Verification items for this drawing (mm, ordinates from the low corner). A direction names the side the tool comes from. Round coordinates to 2 decimals unless told otherwise and drop trailing zeros. Order: outer loops, then holes, each group sorted by start corner. A loop starts at its lowest first (then second) coordinate and runs counter-clockwise, first axis right, second up. Notation, with made-up numbers: (31.25, -9.75) -> (41.25, -9.75) arc R18 ccw to (41.25, 18.25) -> close; hole circle Ø5 at (66.5, -10). An arc over 180 degrees is marked (long way). Use a Markdown table: item, result. Add a question column.
Item 1: Sectioned sample at A-A, the plane z = 61. Record the cut outline in (x, y), and give its area (3 significant figures).
Item 2: Set-up check for the marked faces 1, 2 and 3: record each of +Z, -Z, +X, -X, +Y, -Y from which the full face is reachable in a straight line by a thin tool's end or side.
Item 3: Sectioned sample at D-D, the plane z = 270. Record the cut outline in (x, y), and give its area (3 significant figures).
Item 4: Gauge pin test, flat ends, axial feed: pin 1 Ø4 at (x, y) = (56.5, 411) entering from -Z; pin 2 Ø12 at (x, y) = (221, 991.5) entering from +Z; pin 3 Ø12 at (x, y) = (143.5, 2277.5) entering from +Z; pin 4 Ø4 at (y, z) = (1133, 263.5) entering from -X. Record the tip position at first contact, or that the pin passes through.
Item 5: Sectioned sample at B-B, the plane x = 207.5. Record the cut outline in (y, z).
Item 6: Material ranges on probe 1 along X at (y, z) = (819, 104); probe 2 along Y at (x, z) = (229, 436.5); probe 3 along Z at (x, y) = (203.5, 303), recorded low to high. Write a range as [from, to].
Item 7: Sectioned sample at C-C, the plane y = 1834. Record the cut outline in (x, z), and give its area (3 significant figures).
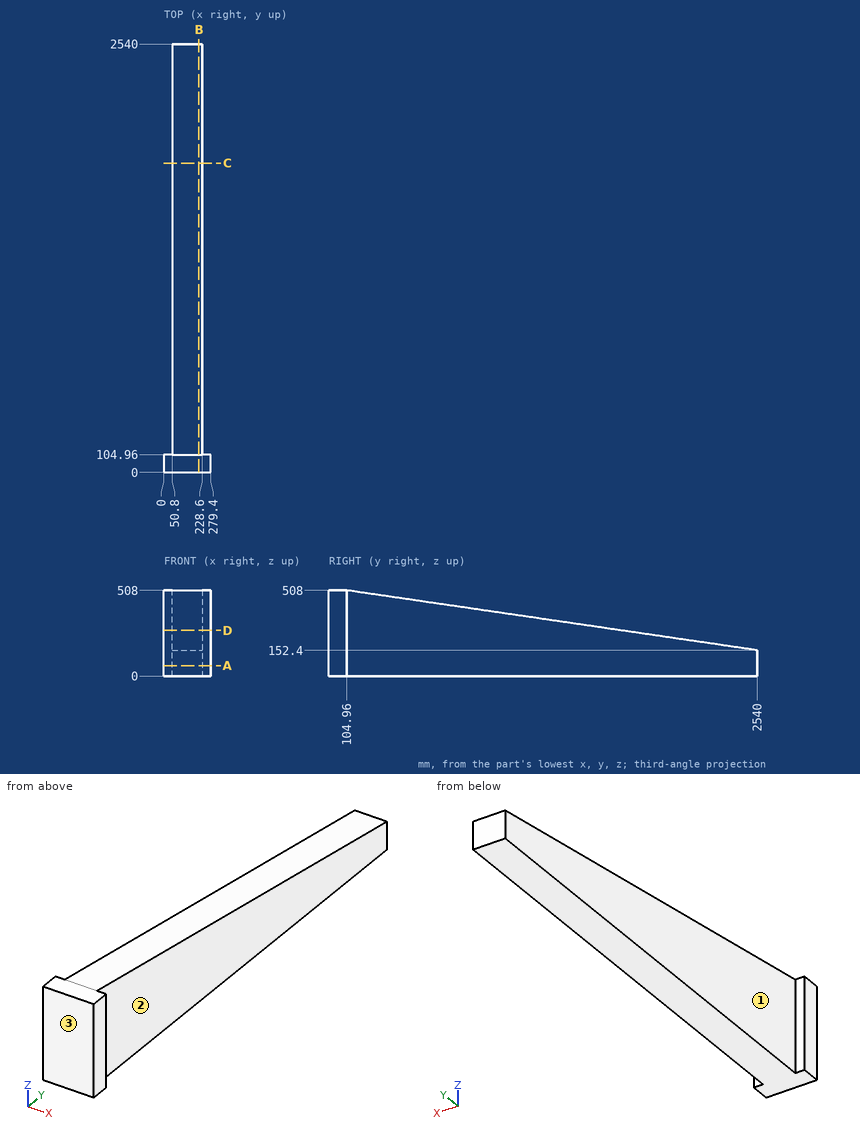
Found:
| question | item | result |
|---|---|---|
| 1 | outline | (0, 0) -> (279.4, 0) -> (279.4, 104.96) -> (228.6, 104.96) -> (228.6, 2540) -> (50.8, 2540) -> (50.8, 104.96) -> (0, 104.96) -> close |
| 1 | area | 462,000 mm2 |
| 2 | face 1 | +Z, -Z, -X, +Y |
| 2 | face 2 | +Z, -Z, +X, +Y |
| 2 | face 3 | +Z, -Z, +X, -X, -Y |
| 3 | outline | (0, 0) -> (279.4, 0) -> (279.4, 104.96) -> (228.6, 104.96) -> (228.6, 1734.71) -> (50.8, 1734.71) -> (50.8, 104.96) -> (0, 104.96) -> close |
| 3 | area | 319,000 mm2 |
| 4 | pin 1 | stops at z = 0 |
| 4 | pin 2 | stops at z = 379.41 |
| 4 | pin 3 | stops at z = 191.61 |
| 4 | pin 4 | stops at x = 50.8 |
| 5 | outline | (0, 0) -> (2540, 0) -> (2540, 152.4) -> (104.96, 508) -> (0, 508) -> close |
| 6 | probe 1 | x = [50.8, 228.6] |
| 6 | probe 2 | y = [0, 104.96] |
| 6 | probe 3 | z = [0, 479.08] |
| 7 | outline | (50.8, 0) -> (228.6, 0) -> (228.6, 255.5) -> (50.8, 255.5) -> close |
| 7 | area | 45,400 mm2 |
